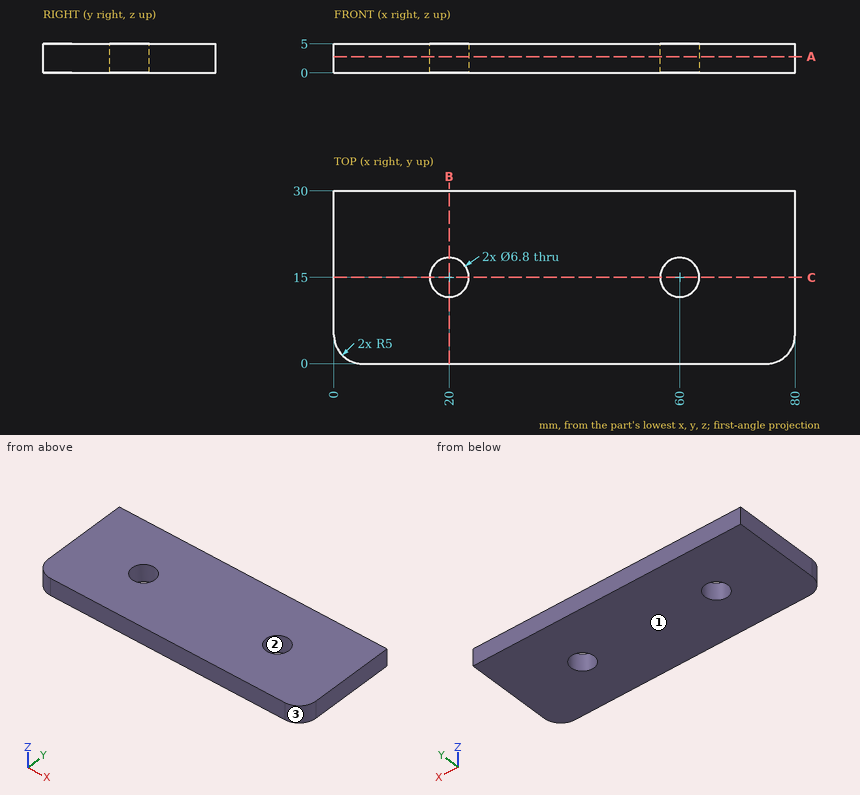
Could you check a few things on this drawing? It's one solid part, dimensions in mm from its lowest x, y, z. Coordinates: 2 decimals unless noted, no trailing zeros. Order: outer loops, then holes, each group sorted by start corner. A loop starts at its lowest first (then second) coordinate and runs counter-clockwise, first axis right, second up.
1. I need wall thicknesses on line 1 (X direction, y = 15.25, z = 1.5); line 2 (Y direction, x = 20, z = 1.5); line 3 (Y direction, x = 61.5, z = 3.15). Which ranges of each line are inside material? Lowest first, please.
2. If we section it at C-C (y = 15): Please give me the cut outline in (x, z), then the cut area to 3 significant figures.
3. If we section it at B-B (x = 20): Please give me the cut outline in (y, z), then the cut area to 3 significant figures.
4. Thinking about a two-plate mould opening in Y: for the marked faces 1, 2 and 3, which applies, +Y half, -Y half, draft (parallel to the pull), parting line (faces both ways), or undercut?
5. If we section it at A-A (z = 2.8): Please give me the cut outline in (x, y).
Entries:
1. line 1: x = 0 to 16.61, 23.39 to 56.61, 63.39 to 80
1. line 2: y = 0 to 11.6, 18.4 to 30
1. line 3: y = 0 to 11.95, 18.05 to 30
2. outline: (0, 0) - (16.6, 0) - (16.6, 5) - (0, 5) - close; (23.4, 0) - (56.6, 0) - (56.6, 5) - (23.4, 5) - close; (63.4, 0) - (80, 0) - (80, 5) - (63.4, 5) - close
2. area: 332 mm2
3. outline: (0, 0) - (11.6, 0) - (11.6, 5) - (0, 5) - close; (18.4, 0) - (30, 0) - (30, 5) - (18.4, 5) - close
3. area: 116 mm2
4. face 1: draft
4. face 2: undercut
4. face 3: -Y half
5. outline: (0, 5) arc R5 ccw to (5, 0) - (75, 0) arc R5 ccw to (80, 5) - (80, 30) - (0, 30) - close; hole circle Ø6.8 at (20, 15); hole circle Ø6.8 at (60, 15)
